Verification items for the finished model (mm, model axes). Face numbers are marked on the shaded views. A direction names the side the tool comes from. Coordinates: 2 decimals unless noted, no trailing zeros. Loops run counter-clockwise (first coordinate to the right, second up) from the corner with the lowest first, then second, coordinate; pieces in that order, holes last. Notation, with made-up numbers: M 45.5,20.25 L 102.5,20.25 A11 cw 102.5,24.25 Z; hole C 52,69.5 d4. An arc over 180 degrees is marked long. Write item = value, one per line. Start each with the question number.
```python
from build123d import *

# Parameters (mm, degrees)
F1_DEPTH = 63.5
F2_DEPTH = 25.4
F3_DEPTH = 7.9375
F5_R     = 6.35


with BuildPart() as f1:
    # F0 (on Front) → F1 (new body, symmetric)
    with BuildSketch(Plane.XZ):
        Polygon((-41.275, 9.525), (-41.275, -9.525), (41.275, -9.525), (41.275, 9.525), (22.225, 9.525), align=None)
    extrude(amount=F1_DEPTH, both=True)

    # F0 (on Front) → F2 (join, symmetric)
    with BuildSketch(Plane.XZ):
        with BuildLine():
            Line((22.225, 9.525), (41.275, 9.525))
            Line((41.275, 9.525), (41.275, 27.0002))
            ThreePointArc((41.275, 27.0002), (45.9246798487, 38.2255201513), (57.15, 42.8752))
            Line((57.15, 42.8752), (60.325, 42.8752))
            Line((60.325, 42.8752), (60.325, 61.9118876984))
            add(Edge.make_bspline(
                [(57.15, 61.9252), (58.2024017722, 61.9212196773), (59.2640962396, 61.9177081997), (60.325, 61.9118876984)],
                knots=[0.7123833019, 0.7123833019, 0.7123833019, 0.7123833019, 0.7293225906, 0.7293225906, 0.7293225906, 0.7293225906], degree=3))
            ThreePointArc((57.15, 61.9252), (32.4542956671, 51.6959043329), (22.225, 27.0002))
            Line((22.225, 27.0002), (22.225, 9.525))
        make_face()
        with BuildLine():
            Line((60.325, 61.9252), (57.15, 61.9252))
            add(Edge.make_bspline(
                [(57.15, 61.9252), (58.2024017722, 61.9212196773), (59.2640962396, 61.9177081997), (60.325, 61.9118876984)],
                knots=[0.7123833019, 0.7123833019, 0.7123833019, 0.7123833019, 0.7293225906, 0.7293225906, 0.7293225906, 0.7293225906], degree=3))
            Line((60.325, 61.9118876984), (60.325, 61.9252))
        make_face()
        Polygon((85.725, 61.9252), (60.325, 61.9252), (60.325, 61.9118876984), (60.325, 42.8752), (85.725, 42.8752), align=None)
    extrude(amount=F2_DEPTH, both=True)

    # F0 (on Front) → F3 (join, symmetric)
    with BuildSketch(Plane.XZ):
        with BuildLine():
            add(Edge.make_bspline(
                [(-41.275, 9.525), (-14.9323567748, 63.0891993642), (12.8911493683, 62.0925928269), (57.15, 61.9252)],
                knots=[0, 0, 0, 0, 0.7123833019, 0.7123833019, 0.7123833019, 0.7123833019], degree=3))
            Line((-41.275, 9.525), (22.225, 9.525))
            Line((22.225, 9.525), (22.225, 27.0002))
            ThreePointArc((22.225, 27.0002), (32.4542956671, 51.6959043329), (57.15, 61.9252))
        make_face()
    extrude(amount=F3_DEPTH, both=True)

    # F0 (on Front) → F4 (revolve)
    with BuildSketch(Plane.XZ):
        Polygon((85.725, 66.675), (85.725, 61.9252), (85.725, 42.8752), (85.725, 38.1), (111.125, 38.1), (111.125, 66.675), align=None)
    revolve(axis=Axis((85.725, 0, 52.3875), (0, 0, 1)))

    # F5
    f5_edges = [f1.edges().sort_by_distance(p)[0] for p in [
        (-41.275, -63.5, 0),
        (41.275, -63.5, 0),
        (41.275, 63.5, 0),
        (-41.275, 63.5, 0),
    ]]
    fillet(f5_edges, radius=F5_R)


solid = f1.part
```
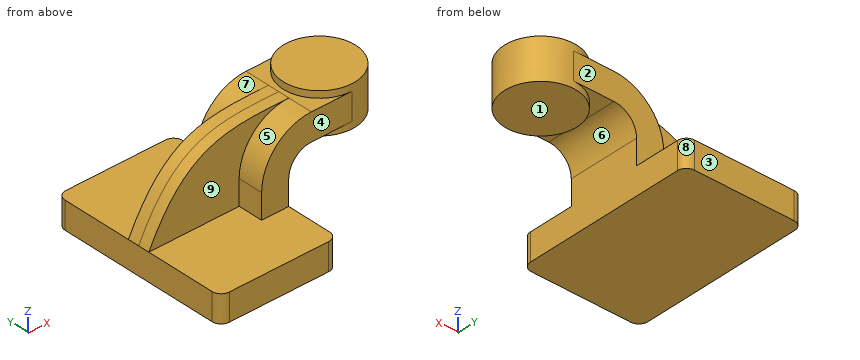
Q1. Scan lines: L1, parallel to Z at x = 73, y = -15.5 (3 decimals); L2, parallel to Z at x = 9, y = -25 (3 decimals); L3, parallel to X at y = 4, z = 0 (3 decimals). Record each from-to range of solid material in increasing order. Write a range as [from, to].
Q2. Sectioned sample at A-A on x = 77.5. Record the cut outline in (y, z) (3 decimals).
Q3. Gauge pin test, flat ends, axial feed: pin 1 (3 mm diameter, centred on x = 18.5, y = 28, fed in from +Z) (3 decimals); pin 2 (19 mm diameter, centred on y = -15.5, z = 17.5, fed in from -X) (3 decimals); pin 3 (3 mm diameter, centred on x = 87.5, z = 54.5, fed in from +Y); pin 4 (8.5 mm diameter, centred on x = 77, y = 8, fed in from -Z). Record the tip position at first contact, or that the pin passes through.
Q4. Mould release check, pull along X, two halves, no side actions. Record for the marked faces 6, 7, 8 and 9: +X half, -X half, draft (parallel to the pull), parting line (faces both ways), or undercut.
Q5. Set-up check for the marked faces 1, 2, 3, 4 and 5: record each of +Z, -Z, +X, -X, +Y, -Y from which the full face is reachable in a straight line by a thin tool's end or side.
Solutions:
q1.L1 = [38.1, 66.675]
q1.L2 = [-9.525, 9.525]
q1.L3 = [-41.275, 41.275]
q2.outline = M -25.4,42.875 L -24.031,42.875 L -24.031,38.1 L 24.031,38.1 L 24.031,42.875 L 25.4,42.875 L 25.4,61.925 L 24.031,61.925 L 24.031,66.675 L -24.031,66.675 L -24.031,61.925 L -25.4,61.925 Z
q3.pin_1 = 9.525
q3.pin_2 = -41.275
q3.pin_3 = 25.4
q3.pin_4 = 38.1
q4.face_6 = undercut
q4.face_7 = -X half
q4.face_8 = +X half
q4.face_9 = draft
q5.face_1 = -Z, +X, +Y, -Y
q5.face_2 = +Z, +X, -X, +Y
q5.face_3 = +Z, -Z, +X, -X, +Y
q5.face_4 = +Z, +X, -X, -Y
q5.face_5 = +Z, -X, -Y
